Geometry check sheet. Reference: the model listing, model coordinates, mm. Give positions to 0.01 mm unless a question says otherwise; leave off trailing zeros. Write each loop counter-clockwise with the first axis right and the second up, starting at its lowest first coordinate (ties: lowest second). Pieces come first, ordered by that corner, then holes. Notation, with made-up numbers: (70, 0) -> (85, 0) arc R21 ccw to (85, 35) -> close; hole circle Ø1 at (-37.75, -31). An arc over 180 degrees is marked (long way). Write item = value, one per line. Start each with the question number.
1. Cross-section at C-C, the plane y = -29.5. Record the cut outline in (x, z), plus the area to 3 significant figures.
2. Cross-section at A-A, the plane z = -44. Record the cut outline in (x, y).
3. Mould release check, pull along X, two halves, no side actions. Record for faces 1 (the flat face through (0, -63, -30.762)), 2 (the flat face through (-31.75, -63, 0)), 3 (the cylindrical face through (0.79, -62.61, -60.78)), 4 (the cylindrical face through (-0.712, -62.611, -63.503)): pulls with the +X half, pulls with the -X half, needs draft (parallel to the pull), parting line crosses it, or undercut.
4. Thickness scan on line 1 along Z through (x, y) = (0, -6); line 2 along X through (y, z) = (-32, -41); line 3 along Z through (x, y) = (4.5, -9). Record the ranges inside material, lowest first.
5. Cross-section at B-B, the plane x = 0. Record the cut outline in (y, z), plus the area to 3 significant figures.
6. Depth check by flat-ended pin: P1, Ø1.5, axis at y = -95.5, z = -34.5, coming from the +X side; P2, Ø3, axis at y = -81.5, z = 18.5, coming from the +X side; P3, Ø10, axis at x = -8, y = -46.5, coming from the -Z side. Enter the tip coordinate at first touch or a pass-through.
```python
from build123d import *

# Parameters (mm, degrees)
F0_W     = 63.5
F0_H     = 63.5
F1_DEPTH = 127
F2_R     = 31.765228
F3_DEPTH = 127
F5_DEPTH = 152.4


with BuildPart() as f1:
    # F0 (on Front) → F1 (new body)
    with BuildSketch(Plane.XZ):
        Rectangle(F0_W, F0_H)
    extrude(amount=F1_DEPTH)

    # F2 (on Front) → F3 (join)
    with BuildSketch(Plane.XZ):
        with Locations((0, -31.745933)):
            Circle(F2_R)
    extrude(amount=F3_DEPTH)

    # F4 (on face) → F5 (cut)
    with BuildSketch(Plane(origin=(0, 0, 0), x_dir=(-1, 0, 0), z_dir=(0, 1, 0))):
        with BuildLine():
            Line((29.699003, -30.762452), (-29.970478, -30.762452))
            ThreePointArc((-29.970478, -30.762452), (-0.135737, -60.78653), (29.699003, -30.762452))
        make_face()
    extrude(amount=-F5_DEPTH, mode=Mode.SUBTRACT)


solid = f1.part
```
Answers:
q1.outline = (-31.75, -30.76) arc R31.77 ccw (long way) to (31.75, -30.76) -> (31.75, 31.75) -> (-31.75, 31.75) -> close; hole (-29.7, -30.76) arc R29.84 ccw (long way) to (29.97, -30.76) -> close
q1.area = 4,210 mm^2
q2.outline = (-29.31, -127) -> (-26.69, -127) -> (-26.69, 0) -> (-29.31, 0) -> close; (26.97, -127) -> (29.31, -127) -> (29.31, 0) -> (26.97, 0) -> close
q3.face_1 = undercut
q3.face_2 = pulls with the -X half
q3.face_3 = undercut
q3.face_4 = parting line crosses it
q4.line_1 = -63.51 to -60.79, -30.76 to 31.75
q4.line_2 = -30.39 to -27.96, 28.23 to 30.39
q4.line_3 = -63.19 to -60.47, -30.76 to 31.75
q5.outline = (-127, -63.51) -> (0, -63.51) -> (0, -60.79) -> (-127, -60.79) -> close; (-127, -30.76) -> (0, -30.76) -> (0, 31.75) -> (-127, 31.75) -> close
q5.area = 8,290 mm^2
q6.P1 = 31.7
q6.P2 = 31.75
q6.P3 = -63.37
